The figure shows three views and two pictorial views of one solid part (mm, origin at its lowest corner). Answer the questions. Coordinates: 2 decimals unless noted, no trailing zeros. Write each loop counter-clockwise with the first axis right and the second up, starting at its lowest first coordinate (ties: lowest second). Pieces come first, ordered by that corner, then holes.
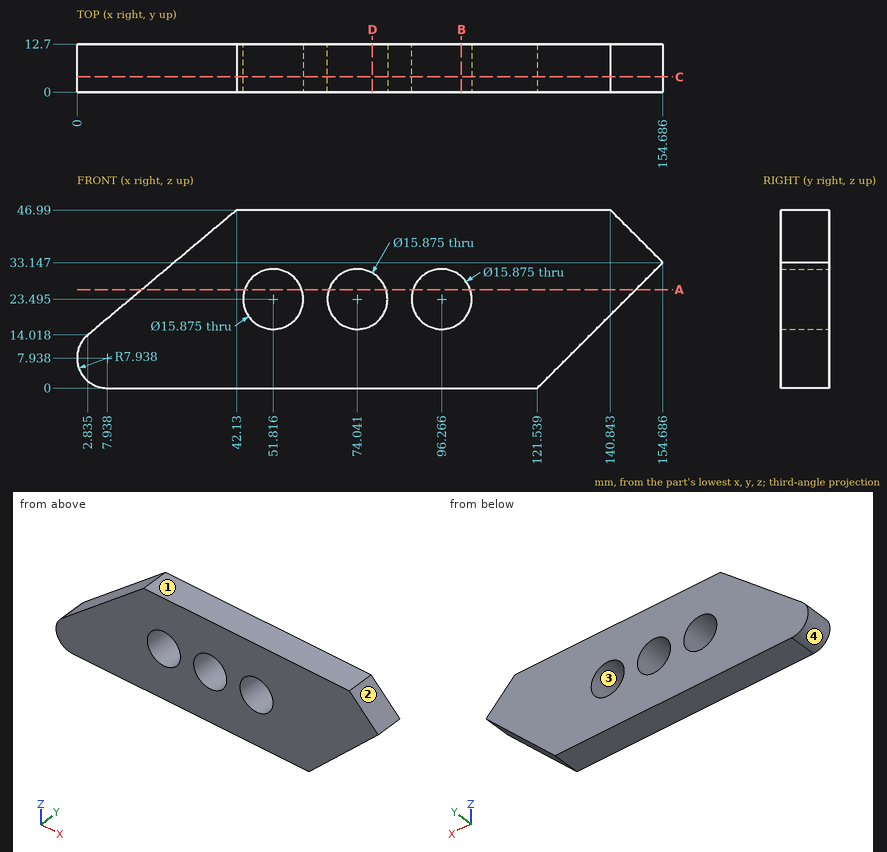
1. Flat-ended cylindrical pins translate along their axes: P1, Ø1, axis at y = 8.5, z = 22.5, coming from the -X side; P2, Ø1, axis at x = 124, y = 11, coming from the -Z side. Find the tip coordinate at first contact, or state that the pin passes through.
Results found:
P1: stops at x = 12.35
P2: stops at z = 1.96
2. Section B-B on x = 101.5 is taken. Give the vertices of the cut face in (y, z).
Results found:
outline: (0, 0) - (12.7, 0) - (12.7, 17.53) - (0, 17.53) - close; (0, 29.46) - (12.7, 29.46) - (12.7, 46.99) - (0, 46.99) - close
3. For a pull along X with two mould halves and no side action, classify the marked faces 1, 2, 3 and 4 as pulls with the +X half, pulls with the -X half, needs draft (parallel to the pull), parting line crosses it, or undercut.
Results found:
face 1: needs draft
face 2: pulls with the +X half
face 3: undercut
face 4: pulls with the -X half
4. Section D-D on x = 78 is taken. Give the vertices of the cut face in (y, z) (1 decimal), then the cut area to 3 significant figures.
Results found:
outline: (0, 0) - (12.7, 0) - (12.7, 16.6) - (0, 16.6) - close; (0, 30.4) - (12.7, 30.4) - (12.7, 47) - (0, 47) - close
area: 422 mm2
5. Section C-C on y = 4 is taken. Give the vertices of the cut face in (x, z) (1 decimal).
Results found:
outline: (2.8, 14) arc R7.9 ccw to (7.9, 0) - (121.5, 0) - (154.7, 33.1) - (140.8, 47) - (42.1, 47) - close; hole circle Ø15.9 at (51.8, 23.5); hole circle Ø15.9 at (74, 23.5); hole circle Ø15.9 at (96.3, 23.5)
6. Section A-A on z = 26 is taken. Give the vertices of the cut face in (x, y) (1 decimal), then the cut area to 3 significant figures.
Results found:
outline: (17.1, 0) - (44.3, 0) - (44.3, 12.7) - (17.1, 12.7) - close; (59.3, 0) - (66.5, 0) - (66.5, 12.7) - (59.3, 12.7) - close; (81.6, 0) - (88.7, 0) - (88.7, 12.7) - (81.6, 12.7) - close; (103.8, 0) - (147.5, 0) - (147.5, 12.7) - (103.8, 12.7) - close
area: 1,080 mm2
7. Find the intervals of material crossed by L1, parallel to Z at x = 89, y = 2 (1 decimal); L2, parallel to X at y = 1.75, z = 26.5 (1 decimal); L3, parallel to Z at x = 68, y = 10 (1 decimal), in increasing order.
Results found:
L1: z = 0 to 20.3, 26.7 to 47
L2: x = 17.7 to 44.5, 59.2 to 66.7, 81.4 to 88.9, 103.6 to 148
L3: z = 0 to 18.3, 28.6 to 47
